Read the model definition and answer for the solid it produces. Units are mm, in the model's axes. A direction names the side the tool comes from. Coordinates: 2 decimals unless noted, no trailing zeros. Write each loop counter-clockwise with the first axis right and the second up, starting at its lowest first coordinate (ties: lowest second). Pieces come first, ordered by that corner, then holes.
Item 1: A tool of negligible diameter and unlimited length cuts with its end or side. For faces 1 (the face through (-3.522, 28.531, -6.216)), 2 (the face through (-5.2, 9.525, 0.1)), 3 (the face through (-7.3, 25.4, -0.2)), 4 (the face through (3.62, 28.53, -6.16)), from which of +Z, -Z, +X, -X, +Y, -Y can it reach the whole face along a straight path? Write none if from no direction.
Item 2: Determine the mould class of faces 5 (the face through (-3.62, 28.53, 6.16)), 6 (the face through (-7.144, 29, 0)), 7 (the face through (-3.86, 4.7, -6.57)) for opening direction Z: released by +Z, released by -Z, zero draft, split by the parting line, or undercut.
Item 3: Section A-A (z = 0) is taken. Give the vertices of the cut face in (x, y) (3 decimals).
Item 4: Each of these flat-tipped pins is pushed along its axis until it touches: P1, Ø1.9, axis at y = 29.5, z = -0.5, coming from the -X side; P2, Ø7.5, axis at x = -1, z = 3.5, coming from the -Y side (3 decimals); P3, Ø5, axis at x = -7.5, z = -11, coming from the +Y side. Where does it stop, or does it pass through?
Item 5: Section D-D (y = 20.5) is taken. Give the vertices of the cut face in (x, z) (3 decimals).
Item 6: Section B-B (y = 5) is taken. Give the vertices of the cut face in (x, z) (3 decimals), then the cut area to 3 significant figures.
Item 7: Straight lines are drawn through the part: probe 1 along X at (y, z) = (26, 0); probe 2 along X at (y, z) = (14, 0) (3 decimals); probe 3 along Y at (x, z) = (13, -1.5). For each, find the intervals that lie inside material, in ascending order.
Item 8: Section C-C (x = -4.5) is taken. Give the vertices of the cut face in (y, z) (3 decimals), then the cut area to 3 significant figures.
from build123d import *

# Parameters (mm, degrees)
SKETCH1_W           = 10.8331
SKETCH1_H           = 25.4
CUT_EXTRUDE1_DEPTH  = 9.525
BOSS_EXTRUDE1_DEPTH = 6.35
SKETCH5_R           = 5.0419
CUT_EXTRUDE2_DEPTH  = 34.89972345


with BuildPart() as part:
    # Sketch1 → Revolve1 (revolve)
    with BuildSketch(Plane.XY, mode=Mode.PRIVATE) as revolve1_sk:
        with Locations((10.45845, 12.7)):
            Rectangle(SKETCH1_W, SKETCH1_H)
    revolve(revolve1_sk.sketch.rotate(Axis((0, 0, 0), (0, 1, 0)), 90), axis=Axis((0, 0, 0), (0, 1, 0)))

    # Sketch3 → Cut-Extrude1 (cut)
    with BuildSketch(Plane.XZ):
        Polygon((7.62, -4.399409051), (7.62, 4.399409051), (0, 8.798818102), (-7.62, 4.399409051), (-7.62, -4.399409051), (0, -8.798818102), align=None)
    extrude(amount=-CUT_EXTRUDE1_DEPTH, mode=Mode.SUBTRACT)

    # Sketch4 → Boss-Extrude1 (add)
    with BuildSketch(Plane(origin=(0, 25.4, 0), x_dir=(1, 0, 0), z_dir=(0, 1, 0))):
        Polygon((0, 8.248891971), (-7.14375, 4.124445986), (-7.14375, -4.124445986), (0, -8.248891971), (7.14375, -4.124445986), (7.14375, 4.124445986), align=None)
    extrude(amount=BOSS_EXTRUDE1_DEPTH)

    # Sketch5 → Cut-Extrude2 (cut, through all)
    with BuildSketch(Plane.XZ.offset(-25.4)):
        with Locations(Location((0, 0, 0), (0, 0, 270))):
            Circle(SKETCH5_R)
    extrude(amount=-CUT_EXTRUDE2_DEPTH, mode=Mode.SUBTRACT)


solid = part.part
Established:
1. face 1: -Z, -X, +Y
1. face 2: -Y
1. face 3: +Y
1. face 4: -Z, +X, +Y
2. face 5: released by +Z
2. face 6: zero draft
2. face 7: undercut
3. outline: (-15.875, 0) - (-7.62, 0) - (-7.62, 9.525) - (-5.042, 9.525) - (-5.042, 31.75) - (-7.144, 31.75) - (-7.144, 25.4) - (-15.875, 25.4) - close; (5.042, 9.525) - (7.62, 9.525) - (7.62, 0) - (15.875, 0) - (15.875, 25.4) - (7.144, 25.4) - (7.144, 31.75) - (5.042, 31.75) - close
4. P1: stops at x = -7.14
4. P2: stops at y = 9.525
4. P3: stops at y = 25.4
5. outline: circle Ø31.75 at (0, 0); hole circle Ø10.084 at (0, 0)
6. outline: circle Ø31.75 at (0, 0); hole (-7.62, -4.399) - (0, -8.799) - (7.62, -4.399) - (7.62, 4.399) - (0, 8.799) - (-7.62, 4.399) - close
6. area: 591 mm2
7. probe 1: x = -7.14 to -5.04, 5.04 to 7.14
7. probe 2: x = -15.875 to -5.042, 5.042 to 15.875
7. probe 3: y = 0 to 25.4
8. outline: (0, -15.224) - (25.4, -15.224) - (25.4, -5.651) - (31.75, -5.651) - (31.75, -2.274) - (9.525, -2.274) - (9.525, -6.201) - (0, -6.201) - close; (0, 6.201) - (9.525, 6.201) - (9.525, 2.274) - (31.75, 2.274) - (31.75, 5.651) - (25.4, 5.651) - (25.4, 15.224) - (0, 15.224) - close
8. area: 626 mm2
